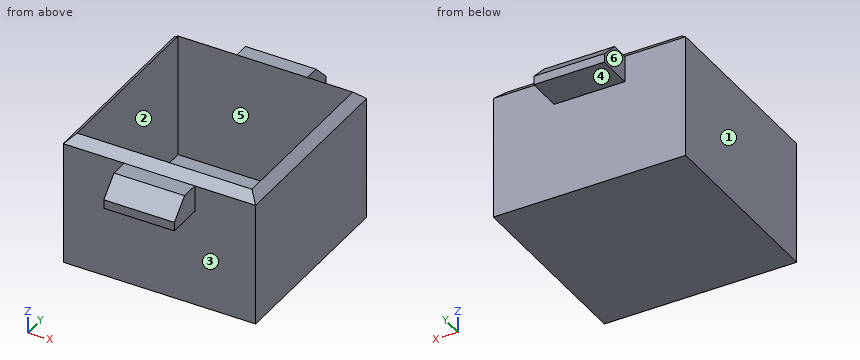
```python
from build123d import *

# Parameters (mm, degrees)
F0_W         = 54.5
F0_H         = 20
F1_DEPTH     = 54.5
F2_DEPTH     = 20
F3_T         = -2.5
F4_W         = 10
F4_H         = 7.5
F5_DEPTH     = 10
F6_W         = 10
F6_H         = 7.5
F7_DEPTH     = 10
F8_T1_DEPTH  = 45.7168298797
F8_T3_DEPTH  = 80.2168298797
F8_T8_DEPTH  = 80.2168298797
F8_T14_DEPTH = 80.2168298797
F8_T21_DEPTH = 80.2168298797
F8_T27_DEPTH = 80.2168298797
F8_T33_DEPTH = 80.2168298797
F8_T40_DEPTH = 80.2168298797


# Not quite as in the source:
# - a fillet or chamfer that OpenCascade refuses, or shapes differently, is made with other operations: its cross-section is extruded or revolved along the edge and cut away or added


with BuildPart() as f1:
    # F0 (on Front) → F1 (new body)
    with BuildSketch(Plane.XZ):
        Rectangle(F0_W, F0_H)
    extrude(amount=F1_DEPTH)

    # F2 (add): a face of the model
    f2_faces = [f1.faces().sort_by_distance(p)[0] for p in [
        (0, -27.25, 10),
    ]]
    extrude(f2_faces, amount=F2_DEPTH)

    # F3
    f3_openings = [f1.faces().sort_by_distance(p)[0] for p in [
        (0, -27.25, 30),
    ]]
    offset(amount=F3_T, openings=f3_openings)

    # F4 (on face) → F5 (join)
    with BuildSketch(Plane.XZ.offset(54.5)):
        with Locations((-5, 21.25)):
            Rectangle(F4_W, F4_H)
        with Locations((5, 21.25)):
            Rectangle(F4_W, F4_H)
    extrude(amount=F5_DEPTH)

    # F6 (on face) → F7 (join)
    with BuildSketch(Plane(origin=(0, 0, 0), x_dir=(-1, 0, 0), z_dir=(0, 1, 0))):
        with Locations((-5, 21.25)):
            Rectangle(F6_W, F6_H)
        with Locations((5, 21.25)):
            Rectangle(F6_W, F6_H)
    extrude(amount=F7_DEPTH)

    # F8: chamfer of 5 on 6 edges, made by hand

    # F8_s2 → F8_t1 (cut)
    with BuildSketch(Plane.YZ.offset(-22.8584149398)):
        Polygon((5, 25), (10, 20), (10, 25), align=None)
        Polygon((-59.5, 25), (-64.5, 20), (-64.5, 25), align=None)
    extrude(amount=F8_T1_DEPTH, mode=Mode.SUBTRACT)

    # F8_s4 → F8_t3 (cut)
    with BuildSketch(Plane.XZ.offset(-12.8584149398)):
        Polygon((-22.25, 30), (-27.25, 25), (-27.25, 30), align=None)
        Polygon((27.25, 25), (22.25, 30), (27.25, 30), align=None)
    extrude(amount=F8_T3_DEPTH, mode=Mode.SUBTRACT)


with BuildPart() as f8_tool6:
    # F8_s7 → F8_t8 (new body)
    with BuildSketch(Plane.YZ.offset(40.1084149398)):
        Polygon((-5, 30), (0, 25), (0, 30), align=None)
    extrude(amount=-F8_T8_DEPTH)

    split(bisect_by=Plane.YZ.offset(10), keep=Keep.TOP)

    split(bisect_by=Plane.XY.offset(25), keep=Keep.TOP)


with BuildPart() as f1_1:
    add(f1.part)

    # F8_t5: cut F8_tool6
    add(f8_tool6.part, mode=Mode.SUBTRACT)


with BuildPart() as f8_tool12:
    # F8_s13 → F8_t14 (new body)
    with BuildSketch(Plane.YZ.offset(40.1084149398)):
        Polygon((-5, 30), (0, 25), (0, 30), align=None)
    extrude(amount=-F8_T14_DEPTH)

    split(bisect_by=Plane.YZ.offset(10), keep=Keep.BOTTOM)

    split(bisect_by=Plane.XY.offset(25), keep=Keep.TOP)

    split(bisect_by=Plane.YZ.offset(-10), keep=Keep.TOP)


with BuildPart() as f1_2:
    add(f1_1.part)

    # F8_t11: cut F8_tool12
    add(f8_tool12.part, mode=Mode.SUBTRACT)


with BuildPart() as f8_tool19:
    # F8_s20 → F8_t21 (new body)
    with BuildSketch(Plane.YZ.offset(40.1084149398)):
        Polygon((-5, 30), (0, 25), (0, 30), align=None)
    extrude(amount=-F8_T21_DEPTH)

    split(bisect_by=Plane.XY.offset(25), keep=Keep.TOP)

    split(bisect_by=Plane.YZ.offset(-10), keep=Keep.BOTTOM)


with BuildPart() as f1_3:
    add(f1_2.part)

    # F8_t18: cut F8_tool19
    add(f8_tool19.part, mode=Mode.SUBTRACT)


with BuildPart() as f8_tool25:
    # F8_s26 → F8_t27 (new body)
    with BuildSketch(Plane.YZ.offset(40.1084149398)):
        Polygon((-54.5, 25), (-49.5, 30), (-54.5, 30), align=None)
    extrude(amount=-F8_T27_DEPTH)

    split(bisect_by=Plane.YZ.offset(10), keep=Keep.TOP)

    split(bisect_by=Plane.XY.offset(25), keep=Keep.TOP)


with BuildPart() as f1_4:
    add(f1_3.part)

    # F8_t24: cut F8_tool25
    add(f8_tool25.part, mode=Mode.SUBTRACT)


with BuildPart() as f8_tool31:
    # F8_s32 → F8_t33 (new body)
    with BuildSketch(Plane.YZ.offset(40.1084149398)):
        Polygon((-54.5, 25), (-49.5, 30), (-54.5, 30), align=None)
    extrude(amount=-F8_T33_DEPTH)

    split(bisect_by=Plane.YZ.offset(-10), keep=Keep.TOP)

    split(bisect_by=Plane.YZ.offset(10), keep=Keep.BOTTOM)

    split(bisect_by=Plane.XY.offset(25), keep=Keep.TOP)


with BuildPart() as f1_5:
    add(f1_4.part)

    # F8_t30: cut F8_tool31
    add(f8_tool31.part, mode=Mode.SUBTRACT)


with BuildPart() as f8_tool38:
    # F8_s39 → F8_t40 (new body)
    with BuildSketch(Plane.YZ.offset(40.1084149398)):
        Polygon((-54.5, 25), (-49.5, 30), (-54.5, 30), align=None)
    extrude(amount=-F8_T40_DEPTH)

    split(bisect_by=Plane.YZ.offset(-10), keep=Keep.BOTTOM)

    split(bisect_by=Plane.XY.offset(25), keep=Keep.TOP)


with BuildPart() as f1_6:
    add(f1_5.part)

    # F8_t37: cut F8_tool38
    add(f8_tool38.part, mode=Mode.SUBTRACT)


solid = f1_6.part
```
The model under review builds one solid part; all positions refer to its coordinate system, in mm. Face numbers are marked on the shaded views. A direction names the side the tool comes from. Round coordinates to 2 decimals unless told otherwise and drop trailing zeros. Write each loop counter-clockwise with the first axis right and the second up, starting at its lowest first coordinate (ties: lowest second). Pieces come first, ordered by that corner, then holes. Notation, with made-up numbers: M 74.25,0 L 95.25,0 A31 cw 95.25,27 Z; hole C 26,13 d9. An arc over 180 degrees is marked long. Use CSV: the item, a comma, the result in double quotes. Start each with the question number.
(1) We need section C-C, the plane x = -15. State the section outline as (y, z) points, then the cut area to 3 significant figures.
(2) We need section A-A, the plane z = -2. State the section outline as (x, y) points, then the cut area to 3 significant figures.
(3) Clearance check with flat-ended pins moving along their axes: P1, Ø10, axis at x = 2.5, z = 8, coming from the +Y side; P2, Ø2, axis at x = 5.5, z = 1, coming from the -Y side; P3, Ø1.5, axis at x = 1.5, y = -56, coming from the +Z side. State where each tip first meets the part, or that it passes through.
(4) We need section D-D, the plane z = 21. State the section outline as (x, y) points.
(5) For line 1 along X through (y, z) = (-35.5, 9.5); line 2 along Y through (x, z) = (24.5, 24.5); line 3 along X through (y, z) = (-61, 19.5), list the stretches that pass through material, from the lowest coordinate up.
(6) We need section B-B, the plane y = -49.5. State the section outline as (x, z) points.
(7) The part is to be moulded in two halves that separate along X. For the marked faces 1, 2 and 3, say which applies: +X half, -X half, draft (parallel to the pull), parting line (faces both ways), or undercut.
(8) Tool access review of the marked faces 4, 5 and 6: name each direction out of +Z, -Z, +X, -X, +Y, -Y from which nothing blocks a thin tool from reaching the whole face with its end or side.
Findings:
1,outline,"M -54.5,-10 L 0,-10 L 0,25 L -2.5,27.5 L -2.5,-7.5 L -52,-7.5 L -52,27.5 L -54.5,25 Z"
1,area,"305 mm^2"
2,outline,"M -27.25,-54.5 L 27.25,-54.5 L 27.25,0 L -27.25,0 Z; hole M -24.75,-52 L 24.75,-52 L 24.75,-2.5 L -24.75,-2.5 Z"
2,area,"520 mm^2"
3,P1,"y = 0"
3,P2,"y = -54.5"
3,P3,"z = 25"
4,outline,"M -27.25,-54.5 L -10,-54.5 L -10,-63.5 L 10,-63.5 L 10,-54.5 L 27.25,-54.5 L 27.25,0 L 10,0 L 10,9 L -10,9 L -10,0 L -27.25,0 Z; hole M -24.75,-52 L 24.75,-52 L 24.75,-2.5 L -24.75,-2.5 Z"
5,line 1,"-27.25 to -24.75, 24.75 to 27.25"
5,line 2,"-54.5 to -52, -2.5 to 0"
5,line 3,"-10 to 10"
6,outline,"M -27.25,-10 L 27.25,-10 L 27.25,25 L 24.75,27.5 L 24.75,-7.5 L -24.75,-7.5 L -24.75,27.5 L -27.25,25 Z"
7,face 1,"-X half"
7,face 2,"undercut"
7,face 3,"draft"
8,face 4,"-Z, +X, -X, +Y"
8,face 5,"+Z"
8,face 6,"+Z, -Z, -X, +Y"
